```python
from build123d import *

# Parameters (mm, degrees)
F0_W      = 140
F0_H      = 30
F1_DEPTH  = 5
F2_W      = 10
F2_H      = 5
F3_DEPTH  = 5
F2_H_2    = 9
F5_W      = 5
F5_H      = 8
F6_DEPTH  = 25
F7_W      = 120
F7_H      = 2
F8_DEPTH  = 5
F9_W      = 115
F9_H      = 1
F10_DEPTH = 25
F11_W     = 4
F11_H     = 33
F12_DEPTH = 5


# Not quite as in the source:
# - a feature names something its author has since deleted; it is built from what else it names


with BuildPart() as f1:
    # F0 (on Top) → F1 (new body)
    with BuildSketch(Plane.XY):
        Rectangle(F0_W, F0_H)
    extrude(amount=F1_DEPTH)


with BuildPart() as f3:
    # F2 (on face) → F3 (new body)
    with BuildSketch(Plane.XY.offset(5)):
        with Locations((65, 17.5)):
            Rectangle(F2_W, F2_H)
    extrude(amount=-F3_DEPTH)


with BuildPart() as f3b:
    # F2 (on face) → F3, piece 2 (new body)
    with BuildSketch(Plane.XY.offset(5)):
        with Locations((-65, 17.5)):
            Rectangle(F2_W, F2_H)
    extrude(amount=-F3_DEPTH)


with BuildPart() as f3c:
    # F2 (on face) → F3, piece 3 (new body)
    with BuildSketch(Plane.XY.offset(5)):
        with Locations((-65, -19.5)):
            Rectangle(F2_W, F2_H_2)
    extrude(amount=-F3_DEPTH)


with BuildPart() as f3d:
    # F2 (on face) → F3, piece 4 (new body)
    with BuildSketch(Plane.XY.offset(5)):
        with Locations((65, -19.5)):
            Rectangle(F2_W, F2_H_2)
    extrude(amount=-F3_DEPTH)


with BuildPart() as f3b_1:
    add(f3b.part)

    # F4: union F3, F3c, F3d, F1
    add(f3.part)
    add(f3c.part)
    add(f3d.part)
    add(f1.part)

    # F5 (on face) → F6 (cut)
    with BuildSketch(Plane.XY.offset(5)):
        with Locations((57.5, 11)):
            Rectangle(F5_W, F5_H)
    extrude(amount=-F6_DEPTH, mode=Mode.SUBTRACT)

    # F7 (on face) → F8 (join)
    with BuildSketch(Plane.XY.offset(5)):
        with Locations((0, -16)):
            Rectangle(F7_W, F7_H)
    extrude(amount=-F8_DEPTH)

    # F9 (on face) → F10 (cut)
    with BuildSketch(Plane.XY.offset(5)):
        with Locations((-2.5, 14.5)):
            Rectangle(F9_W, F9_H)
    extrude(amount=-F10_DEPTH, mode=Mode.SUBTRACT)

    # F11 (on Top) → F12 (join)
    with BuildSketch(Plane.XY):
        with Locations((-72, -2.5)):
            Rectangle(F11_W, F11_H)
        with Locations((72, -2.5)):
            Rectangle(F11_W, F11_H)
    extrude(amount=F12_DEPTH)


solid = f3b_1.part
```
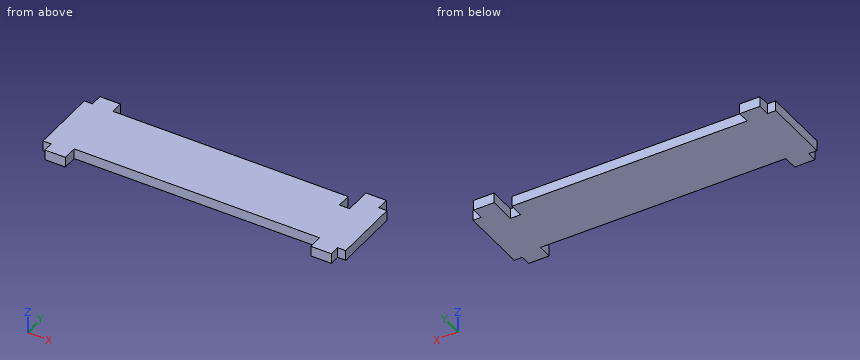
Can you work these out from the model? Positions are in its coordinate system, mm. Give positions to 0.01 mm unless a question says otherwise; leave off trailing zeros. Order: outer loops, then holes, each group sorted by start corner. A loop starts at its lowest first (then second) coordinate and runs counter-clockwise, first axis right, second up. Notation, with made-up numbers: M -33.75,68 L 10.25,68 A12 ccw 10.25,82 Z; hole C 32.5,-2 d11. An arc over 180 degrees is marked long. Write item = value, one per line. Start each with the question number.
Q1. Suppose I cut it at B-B (x = 27). Write out the boundary of the cut face in (y, z).
Q2. Will these pins go through, and if not, where does the flat tip stop? pin 1 Ø1.5 at (x, z) = (58.5, 1.5) entering from +Y; pin 2 Ø1.5 at (y, z) = (16, 2.5) entering from +X; pin 3 Ø1.2 at (x, z) = (72.5, 3) entering from +Y.
Q3. Suppose I cut it at A-A (z = 1). Write out the boundary of the cut face in (x, y), plus the area to 3 significant figures.
Q4. I need wall thicknesses on probe 1 along X at (y, z) = (15.5, 0.75); probe 2 along X at (y, z) = (-18, 3.95); probe 3 along Y at (x, z) = (24.5, 1.3). Which ranges of each line are inside material? Lowest first, please. Write a range as [from, to].
Check result:
q1.outline = M -17,0 L 14,0 L 14,5 L -17,5 Z
q2.pin_1 = 7
q2.pin_2 = 70
q2.pin_3 = 14
q3.outline = M -74,-19 L -70,-19 L -70,-24 L -60,-24 L -60,-17 L 60,-17 L 60,-24 L 70,-24 L 70,-19 L 74,-19 L 74,14 L 70,14 L 70,20 L 60,20 L 60,7 L 55,7 L 55,14 L -60,14 L -60,20 L -70,20 L -70,14 L -74,14 Z
q3.area = 4,830 mm2
q4.probe_1 = [-70, -60], [60, 70]
q4.probe_2 = [-74, -60], [60, 74]
q4.probe_3 = [-17, 14]
